from build123d import *

# Parameters (mm, degrees)
ESBO_O1_W                = 310
ESBO_O1_H                = 320
RESSALTO_EXTRUS_O1_DEPTH = 35
CHANFRO1_SIZE            = 10


with BuildPart() as part:
    # Esboço1 → Ressalto-extrusão1 (new body)
    with BuildSketch(Plane.XY):
        with Locations((-200, -190)):
            Rectangle(ESBO_O1_W, ESBO_O1_H)
    extrude(amount=RESSALTO_EXTRUS_O1_DEPTH)

    # Chanfro1
    chanfro1_edges = [part.edges().sort_by_distance(p)[0] for p in [
        (-355, -190, 35),
        (-45, -190, 35),
        (-355, -190, 0),
        (-45, -190, 0),
    ]]
    chamfer(chanfro1_edges, length=CHANFRO1_SIZE)


solid = part.part
Geometry: final body of the model. Coordinates: model frame, mm. Round coordinates to 2 decimals unless told otherwise and drop trailing zeros. Loops run counter-clockwise (first coordinate to the right, second up) from the corner with the lowest first, then second, coordinate; pieces in that order, holes last. Notation, with made-up numbers: M -28.75,-38.5 L 7.25,-38.5 A21 cw 7.25,-20.5 Z; hole C 2,-20 d5. An arc over 180 degrees is marked long. Put each result on its own line as item: value. Start each with the question number.
(1) Section query A-A (y = -119.5). Return loops of the section in (x, z), then the cut area to 4 significant figures.
(2) Material intervals for line 1 along X through (y, z) = (-76.5, 26.5); line 2 along X through (y, z) = (-310, 29.5), sorted ascending. Write a range as [from, to].
(3) Section query B-B (z = 6). Return loops of the section in (x, y).
Findings below:
1. outline: M -355,10 L -345,0 L -55,0 L -45,10 L -45,25 L -55,35 L -345,35 L -355,25 Z
1. area: 10,650 mm2
2. line 1: x = [-353.5, -46.5]
2. line 2: x = [-350.5, -49.5]
3. outline: M -351,-350 L -49,-350 L -49,-30 L -351,-30 Z
